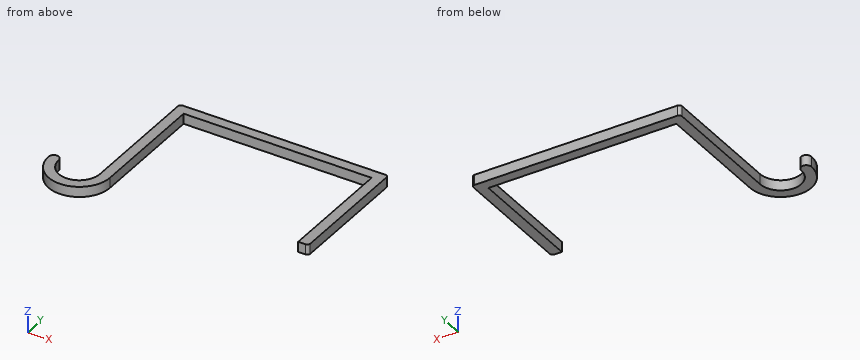
from build123d import *

# Parameters (mm, degrees)
F2_DEPTH = 7


with BuildPart() as f2:
    # F1 (on Top) → F2 (new body)
    with BuildSketch(Plane.XY):
        with BuildLine():
            ThreePointArc((14, 0), (0, -14), (-14, 0))
            ThreePointArc((-14, 0), (-17.5, 3.5), (-21, 0))
            ThreePointArc((-21, 0), (0, -21), (21, 0))
            Line((21, 0), (21, 80))
            Line((21, 80), (149.2, 80))
            Line((149.2, 80), (149.2, 0))
            Line((149.2, 0), (154.2, 0))
            ThreePointArc((154.2, 0), (155.6142135624, 0.5857864376), (156.2, 2))
            Line((156.2, 2), (156.2, 85))
            ThreePointArc((156.2, 85), (155.6142135624, 86.4142135624), (154.2, 87))
            Line((154.2, 87), (16, 87))
            ThreePointArc((16, 87), (14.5857864376, 86.4142135624), (14, 85))
            Line((14, 85), (14, 0))
        make_face()
    extrude(amount=F2_DEPTH)


solid = f2.part
Here's how the part is built. I have some questions about the finished solid (model axes, mm). Give positions to 0.01 mm unless a question says otherwise; leave off trailing zeros. Loops run counter-clockwise (first coordinate to the right, second up) from the corner with the lowest first, then second, coordinate; pieces in that order, holes last. Notation, with made-up numbers: (17.25, 89) -> (58.25, 89) arc R13 ccw to (58.25, 93) -> close; hole circle Ø8 at (-16.5, -19.5). An arc over 180 degrees is marked (long way). One line per item, written item: value.
Q1. I'm going to push flat-ended pins straight in: pin 1 Ø4 at (x, z) = (58.5, 3.5) entering from -Y; pin 2 Ø2.5 at (x, z) = (151.5, 2) entering from -Y; pin 3 Ø1.5 at (y, z) = (59.5, 1) entering from -X. Where does each tip first touch, or does it pass through?
Answers follow:
pin 1: y = 80
pin 2: y = 0
pin 3: x = 14
Q2. Suppose I cut it at C-C on x = 48. Please give me the cut outline in (y, z), then the cut area to 3 significant figures.
Answers follow:
outline: (80, 0) -> (87, 0) -> (87, 7) -> (80, 7) -> close
area: 49.0 mm^2
Q3. If I drill on line 1 along X through (y, z) = (21, 6); line 2 along X through (y, z) = (3, 5); line 3 along X through (y, z) = (82, 1.5), over which ranges is the centre line in solid material (lowest first)?
Answers follow:
line 1: 14 to 21, 149.2 to 156.2
line 2: -19.3 to -15.7, 14 to 21, 149.2 to 156.2
line 3: 14 to 156.2
Q4. Suppose I cut it at D-D on x = -17.5. Please give me the cut outline in (y, z), then the cut area to 3 significant figures.
Answers follow:
outline: (-11.61, 0) -> (3.5, 0) -> (3.5, 7) -> (-11.61, 7) -> close
area: 106 mm^2
Q5. Suppose I cut it at B-B on z = 4.5. Please give me the cut outline in (x, y).
Answers follow:
outline: (-21, 0) arc R21 ccw to (21, 0) -> (21, 80) -> (149.2, 80) -> (149.2, 0) -> (154.2, 0) arc R2 ccw to (156.2, 2) -> (156.2, 85) arc R2 ccw to (154.2, 87) -> (16, 87) arc R2 ccw to (14, 85) -> (14, 0) arc R14 cw to (-14, 0) arc R3.5 ccw to start
Q6. Suppose I cut it at A-A on y = 71.5. Please give me the cut outline in (x, z).
Answers follow:
outline: (14, 0) -> (21, 0) -> (21, 7) -> (14, 7) -> close; (149.2, 0) -> (156.2, 0) -> (156.2, 7) -> (149.2, 7) -> close
